Here's how the part is built. I have some questions about the finished solid (model axes, mm). Face numbers are marked on the shaded views. Coordinates: 2 decimals unless noted, no trailing zeros. Write each loop counter-clockwise with the first axis right and the second up, starting at its lowest first coordinate (ties: lowest second). Pieces come first, ordered by that corner, then holes.
Item 1: I want a section at A-A (y = 40). Please give me the cut outline in (x, z).
Item 2: If we mould it in two halves opening along X, with no side actions, what happens to the marked faces 1, 2 and 3? For each: pulls with the +X half, pulls with the -X half, needs draft (parallel to the pull), parting line crosses it, or undercut.
Item 3: Please list where these lines run through material, in increasing order: line 1 (Y direction, x = 5, z = 2.3); line 2 (X direction, y = 67.5, z = 1.35); line 3 (Z direction, x = 5, y = 30).
Item 4: I want a section at D-D (y = 2.5). Please give me the cut outline in (x, z), and give its area (3 significant figures).
Item 5: I want a section at B-B (z = 2). Please give me the cut outline in (x, y), and give its area (3 significant figures).
Item 6: I'm going to push flat-ended pins straight in: P1, Ø1.5, axis at x = 2, y = 43.5, coming from the +Z side; P2, Ø1, axis at x = 4, z = 7.5, coming from the +Y side. Where does each tip first touch, or does it pass through?
Item 7: I want a section at C-C (x = 5.75). Please give me the cut outline in (y, z).
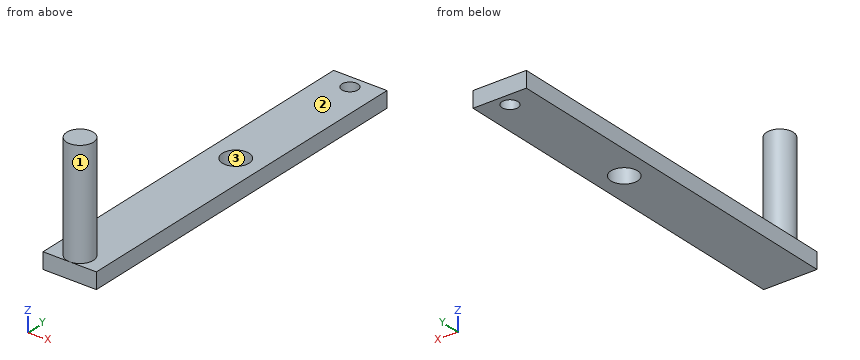
from build123d import *

# Parameters (mm, degrees)
SKETCH1_W           = 10
SKETCH1_H           = 70
BOSS_EXTRUDE1_DEPTH = 3
SKETCH2_R           = 2.5
BOSS_EXTRUDE2_DEPTH = 20
SKETCH4_R           = 1.5
CUT_EXTRUDE1_DEPTH  = 20
SKETCH3_R           = 2.5
CUT_EXTRUDE3_DEPTH  = 20


with BuildPart() as part:
    # Sketch1 → Boss-Extrude1 (new body)
    with BuildSketch(Plane.XY):
        with Locations((5, 35)):
            Rectangle(SKETCH1_W, SKETCH1_H)
    extrude(amount=BOSS_EXTRUDE1_DEPTH)

    # Sketch2 → Boss-Extrude2 (add)
    with BuildSketch(Plane.XY.offset(3)):
        with Locations((5, 2.5)):
            Circle(SKETCH2_R)
    extrude(amount=BOSS_EXTRUDE2_DEPTH)

    # Sketch4 → Cut-Extrude1 (cut)
    with BuildSketch(Plane(origin=(0, 0, 0), x_dir=(-1, 0, 0), z_dir=(0, 0, -1))):
        with Locations((-5, 67.5)):
            Circle(SKETCH4_R)
    extrude(amount=-CUT_EXTRUDE1_DEPTH, mode=Mode.SUBTRACT)

    # Sketch3 → Cut-Extrude3 (cut)
    with BuildSketch(Plane(origin=(0, 0, 0), x_dir=(-1, 0, 0), z_dir=(0, 0, -1))):
        with Locations((-5, 40)):
            Circle(SKETCH3_R)
    extrude(amount=-CUT_EXTRUDE3_DEPTH, mode=Mode.SUBTRACT)


solid = part.part
Answer:
1. outline: (0, 0) - (2.5, 0) - (2.5, 3) - (0, 3) - close; (7.5, 0) - (10, 0) - (10, 3) - (7.5, 3) - close
2. face 1: parting line crosses it
2. face 2: needs draft
2. face 3: undercut
3. line 1: y = 0 to 37.5, 42.5 to 66, 69 to 70
3. line 2: x = 0 to 3.5, 6.5 to 10
3. line 3: z = 0 to 3
4. outline: (0, 0) - (10, 0) - (10, 3) - (7.5, 3) - (7.5, 23) - (2.5, 23) - (2.5, 3) - (0, 3) - close
4. area: 130 mm2
5. outline: (0, 0) - (10, 0) - (10, 70) - (0, 70) - close; hole circle Ø5 at (5, 40); hole circle Ø3 at (5, 67.5)
5. area: 673 mm2
6. P1: stops at z = 3
6. P2: stops at y = 4.95
7. outline: (0, 0) - (37.62, 0) - (37.62, 3) - (4.88, 3) - (4.88, 23) - (0.12, 23) - (0.12, 3) - (0, 3) - close; (42.38, 0) - (66.2, 0) - (66.2, 3) - (42.38, 3) - close; (68.8, 0) - (70, 0) - (70, 3) - (68.8, 3) - close
